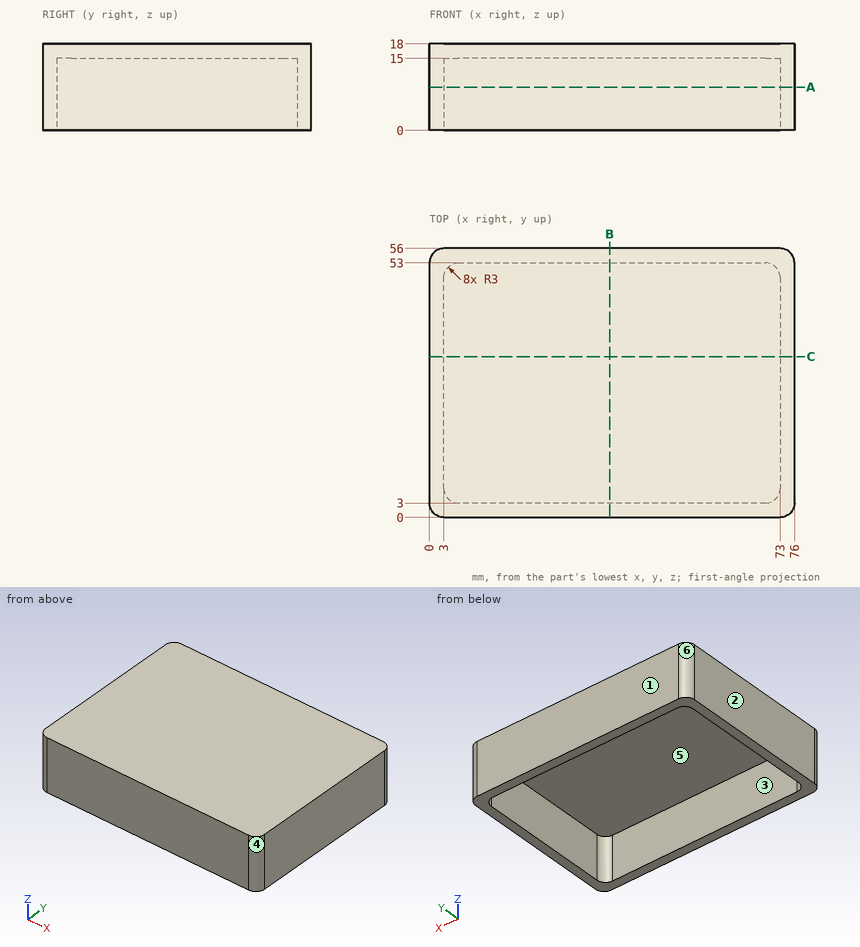
Print and shaded views of the part. All mm, measured from the part's lowest x, y and z. A direction names the side the tool comes from. Coordinates: 2 decimals unless noted, no trailing zeros. Loops run counter-clockwise (first coordinate to the right, second up) from the corner with the lowest first, then second, coordinate; pieces in that order, holes last. Notation, with made-up numbers: (8.5, 35.5) - (23.5, 35.5) arc R17 cw to (23.5, 53.5) - close; hole circle Ø11 at (-8.5, 64). An arc over 180 degrees is marked (long way). Write item = value, one per line. Start each with the question number.
Item 1: Pull direction X, two halves, no side cores. Call the marked faces 1, 2, 3 and 4: +X half, -X half, draft (parallel to the pull), parting line (faces both ways), or undercut.
Item 2: 3-axis set-ups, long thin cutter, end or side, ignore diameter. For the marked faces 5 and 6: which of +Z, -Z, +X, -X, +Y, -Y reach the whole face in a straight line?
Item 3: Wall check: probe 1 along X at (y, z) = (45, 13.5); probe 2 along Y at (x, z) = (10, 9.75); probe 3 along Z at (x, y) = (64.5, 41.5). Give the ranges that are in metal, low to high. Write a range as [from, to].
Item 4: Saw through at B-B, the plane x = 37.5. List the corners of the cut face in (y, z), then the cut area to 3 significant figures.
Item 5: Drop flat-ended pins along their axis: pin 1 Ø10 at (y, z) = (32, 13.5) entering from -X; pin 2 Ø1 at (x, y) = (32.5, 49.5) entering from -Z. Give the stop position or say it passes through.
Item 6: Saw through at A-A, the plane z = 9. List the corners of the cut face in (x, y).
Item 7: Saw through at C-C, the plane y = 33.5. List the corners of the cut face in (x, z), then the cut area to 3 significant figures.
Answers:
q1.face_1 = draft
q1.face_2 = -X half
q1.face_3 = undercut
q1.face_4 = +X half
q2.face_5 = -Z
q2.face_6 = +Z, -Z, -X, +Y
q3.probe_1 = [0, 3], [73, 76]
q3.probe_2 = [0, 3], [53, 56]
q3.probe_3 = [15, 18]
q4.outline = (0, 0) - (3, 0) - (3, 15) - (53, 15) - (53, 0) - (56, 0) - (56, 18) - (0, 18) - close
q4.area = 258 mm2
q5.pin_1 = 0
q5.pin_2 = 15
q6.outline = (0, 3) arc R3 ccw to (3, 0) - (73, 0) arc R3 ccw to (76, 3) - (76, 53) arc R3 ccw to (73, 56) - (3, 56) arc R3 ccw to (0, 53) - close; hole (3, 6) arc R3 ccw to (6, 3) - (70, 3) arc R3 ccw to (73, 6) - (73, 50) arc R3 ccw to (70, 53) - (6, 53) arc R3 ccw to (3, 50) - close
q7.outline = (0, 0) - (3, 0) - (3, 15) - (73, 15) - (73, 0) - (76, 0) - (76, 18) - (0, 18) - close
q7.area = 318 mm2
